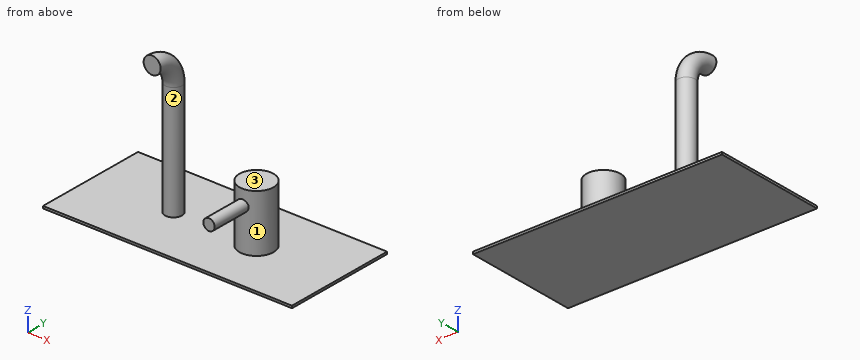
from build123d import *

# Parameters (mm, degrees)
SKETCH_1_W        = 220
SKETCH_1_H        = 100
EXTRUDE_1_DEPTH   = 2
SWEEP_1_PROFILE_R = 7.5
SKETCH_15_R       = 15
EXTRUDE_2_DEPTH   = 50
SKETCH_16_R       = 5
EXTRUDE_3_DEPTH   = 50


with BuildPart() as part:
    # Эскиз1 → Бобышка-Вытянуть1 (new body)
    with BuildSketch(Plane.XY):
        with Locations((110, 50)):
            Rectangle(SKETCH_1_W, SKETCH_1_H)
    extrude(amount=EXTRUDE_1_DEPTH)

    # По траектории1: sweep along a curve in space
    with BuildLine() as sweep_1_path:
        Line((73.333333333, 50, 2), (73.333333333, 50, 102))
        ThreePointArc((73.333333333, 50, 102), (73.333333333, 43.409902577, 117.909902577), (73.333333333, 27.5, 124.5))
    # По траектории1 profile (on start of the path) → По траектории1 (sweep)
    with BuildSketch(Plane(origin=(73.333333333, 50, 2), x_dir=(1, 0, 0), z_dir=(0, 0, 1))):
        Circle(SWEEP_1_PROFILE_R)
    sweep(path=sweep_1_path.line)

    # Эскиз15 → Бобышка-Вытянуть2 (add)
    with BuildSketch(Plane.XY.offset(2)):
        with Locations(Location((146.666666667, 50, 0), (0, 0, 180))):
            Circle(SKETCH_15_R)
    extrude(amount=EXTRUDE_2_DEPTH)

    # Эскиз16 → Бобышка-Вытянуть3 (add)
    with BuildSketch(Plane(origin=(0, 50, 0), x_dir=(-1, 0, 0), z_dir=(0, -1, 0))):
        with Locations(Location((-146.666666667, -38.788976591, 0), (0, 0, 270))):
            Circle(SKETCH_16_R)
    extrude(amount=EXTRUDE_3_DEPTH)


solid = part.part
CAD build for the part. Positions are in the model's coordinates, mm. Face numbers are marked on the shaded views. Give positions to 0.01 mm unless a question says otherwise; leave off trailing zeros. Write each loop counter-clockwise with the first axis right and the second up, starting at its lowest first coordinate (ties: lowest second). Pieces come first, ordered by that corner, then holes. Notation, with made-up numbers: (74.5, 13.25) - (88.5, 13.25) arc R28 ccw to (88.5, 31.25) - close; hole circle Ø1 at (28, -3). An arc over 180 degrees is marked (long way). Answer as CSV lines item,"result".
Q1. Pull direction X, two halves, no side cores. Call the marked faces 1, 2 and 3: released by +X, released by -X, zero draft, split by the parting line, or undercut.
Result set:
face 1,"undercut"
face 2,"undercut"
face 3,"zero draft"
Q2. Drill centre lines: line 1 (Z direction, x = 169.5, y = 95.5); line 2 (X direction, y = 49, z = 113); line 3 (Y direction, x = 153.5, z = 14). Where is each one in solid material? Low to high. Write a range as from..to.
Result set:
line 1,"0..2"
line 2,"66.02..80.65"
line 3,"36.65..63.35"
Q3. Band-saw the part on C-C (z = 76). Give the cut face in (x, y), and give its area (3 significant figures).
Result set:
outline,"circle Ø15 at (73.33, 50)"
area,"177 mm²"
Q4. Flat gauge pins, fed straight in: pin 1 Ø8 at (y, z) = (64, 29) entering from +X; pin 2 Ø16.5 at (x, z) = (76, 127) entering from -Y; pin 3 Ø2 at (x, y) = (64, 88) entering from +Z. Where does each tip first touch, or does it go through?
Result set:
pin 1,"x = 157.85"
pin 2,"y = 27.5"
pin 3,"z = 2"
Q5. Band-saw the part on D-D (y = 77). Give the cut face in (x, z), and give its area (3 significant figures).
Result set:
outline,"(0, 0) - (220, 0) - (220, 2) - (0, 2) - close"
area,"440 mm²"
Q6. Band-saw the part on A-A (y = 9). Give the cut face in (x, z), and give its area (3 significant figures).
Result set:
outline,"(0, 0) - (220, 0) - (220, 2) - (0, 2) - close; circle Ø10 at (146.67, 38.79)"
area,"519 mm²"
Q7. Band-saw the part on B-B (x = 134). Give the cut face in (y, z), and give its area (3 significant figures).
Result set:
outline,"(0, 0) - (100, 0) - (100, 2) - (58.03, 2) - (58.03, 52) - (41.97, 52) - (41.97, 2) - (0, 2) - close"
area,"1,000 mm²"
